```python
from build123d import *

# Parameters (mm, degrees)
BOSS_EXTRUDE1_DEPTH = 2.5
SKETCH2_R           = 2.5
SKETCH2_R_2         = 7.5
CUT_EXTRUDE1_DEPTH  = 63.69968102
SKETCH4_W           = 10
SKETCH4_H           = 10
CUT_EXTRUDE3_DEPTH  = 10


with BuildPart() as part:
    # Sketch1 → Boss-Extrude1 (new, symmetric)
    with BuildSketch(Plane.XY):
        with BuildLine():
            Line((-40, -37.5), (40, -37.5))
            ThreePointArc((40, -37.5), (47.071067812, -34.571067812), (50, -27.5))
            Line((50, -27.5), (50, 27.5))
            ThreePointArc((50, 27.5), (47.071067812, 34.571067812), (40, 37.5))
            Line((40, 37.5), (-40, 37.5))
            ThreePointArc((-40, 37.5), (-47.071067812, 34.571067812), (-50, 27.5))
            Line((-50, 27.5), (-50, -27.5))
            ThreePointArc((-50, -27.5), (-47.071067812, -34.571067812), (-40, -37.5))
        make_face()
    extrude(amount=BOSS_EXTRUDE1_DEPTH, both=True)

    # Sketch2 → Cut-Extrude1 (cut, through all)
    with BuildSketch(Plane.XY.offset(2.5)):
        with Locations((40, 25)):
            Circle(SKETCH2_R)
        with Locations((-40, 25)):
            Circle(SKETCH2_R)
        with Locations((-40, -25)):
            Circle(SKETCH2_R)
        with Locations((40, -25)):
            Circle(SKETCH2_R)
        Circle(SKETCH2_R_2)
    extrude(amount=-CUT_EXTRUDE1_DEPTH, mode=Mode.SUBTRACT)

    # Sketch4 → Cut-Extrude3 (cut)
    with BuildSketch(Plane(origin=(0, 0, -2.5), x_dir=(-1, 0, 0), z_dir=(0, 0, -1))):
        with Locations((45, 0)):
            Rectangle(SKETCH4_W, SKETCH4_H)
        with Locations((-45, 0)):
            Rectangle(SKETCH4_W, SKETCH4_H)
    extrude(amount=-CUT_EXTRUDE3_DEPTH, mode=Mode.SUBTRACT)


solid = part.part
```
Model file for the job. Use its own axes, mm. A direction names the side the tool comes from. Give positions to 0.01 mm unless a question says otherwise; leave off trailing zeros. Write each loop counter-clockwise with the first axis right and the second up, starting at its lowest first coordinate (ties: lowest second). Pieces come first, ordered by that corner, then holes. Notation, with made-up numbers: (57, 86.5) -> (70, 86.5) arc R12 ccw to (70, 101.5) -> close; hole circle Ø3 at (-29.5, 46.5). An arc over 180 degrees is marked (long way). Use CSV: the item, a comma, the result in double quotes. Start each with the question number.
1) Cut at D-D on y = 0. List the corners of the cut face in (x, z), plus the area to 3 significant figures.
2) Cut at B-B on z = 0.5. List the corners of the cut face in (x, y).
3) Drill centre lines: L1, parallel to Y at x = 0, z = 1.4; L2, parallel to X at y = -23.5, z = 1.6; L3, parallel to X at y = 23, z = -1.9. Where is each one in solid material? Low to high.
4) Cut at A-A on x = 6. List the corners of the cut face in (y, z), plus the area to 3 significant figures.
5) Tool access for faces 5 (the flat face through (-45, 5, 0)), 6 (the flat face through (45, 5, 0)), 7 (the flat face through (-50, 16, 0)): list every direction of +Z, -Z, +X, -X, +Y, -Y with a clear straight run to the whole face (end or side of a thin tool).
6) Cut at C-C on y = -25. List the corners of the cut face in (x, z).
7) Pin check, flat tips, straight feed: P1, Ø12, axis at x = 0, y = 0, coming from the +Z side; P2, Ø2.5, axis at y = 0, z = 0.5, coming from the +X side; P3, Ø1.5, axis at y = 2.5, z = -1, coming from the -X side. Stop position of each tip, or through.
8) Two-plate mould, pull along Y, no slides. Class faces 1 (the cylindrical face through (-46.99, 34.65, 0.04)), 2 (the cylindrical face through (46.99, -34.65, 0.04)), 3 (the cylindrical face through (-38.66, -22.89, 0.04)), 4 (the flat face through (-1, 9, 2.5)): released by +Y, released by -Y, zero draft, split by the parting line, or undercut.
Final values:
1,outline,"(-40, -2.5) -> (-7.5, -2.5) -> (-7.5, 2.5) -> (-40, 2.5) -> close; (7.5, -2.5) -> (40, -2.5) -> (40, 2.5) -> (7.5, 2.5) -> close"
1,area,"325 mm2"
2,outline,"(-50, -27.5) arc R10 ccw to (-40, -37.5) -> (40, -37.5) arc R10 ccw to (50, -27.5) -> (50, -5) -> (40, -5) -> (40, 5) -> (50, 5) -> (50, 27.5) arc R10 ccw to (40, 37.5) -> (-40, 37.5) arc R10 ccw to (-50, 27.5) -> (-50, 5) -> (-40, 5) -> (-40, -5) -> (-50, -5) -> close; hole circle Ø5 at (-40, -25); hole circle Ø5 at (-40, 25); hole circle Ø15 at (0, 0); hole circle Ø5 at (40, -25); hole circle Ø5 at (40, 25)"
3,L1,"y = -37.5 to -7.5, 7.5 to 37.5"
3,L2,"x = -50 to -42, -38 to 38, 42 to 50"
3,L3,"x = -50 to -41.5, -38.5 to 38.5, 41.5 to 50"
4,outline,"(-37.5, -2.5) -> (-4.5, -2.5) -> (-4.5, 2.5) -> (-37.5, 2.5) -> close; (4.5, -2.5) -> (37.5, -2.5) -> (37.5, 2.5) -> (4.5, 2.5) -> close"
4,area,"330 mm2"
5,face 5,"+Z, -Z, -X"
5,face 6,"+Z, -Z, +X"
5,face 7,"+Z, -Z, -X, +Y, -Y"
6,outline,"(-50, -2.5) -> (-42.5, -2.5) -> (-42.5, 2.5) -> (-50, 2.5) -> close; (-37.5, -2.5) -> (37.5, -2.5) -> (37.5, 2.5) -> (-37.5, 2.5) -> close; (42.5, -2.5) -> (50, -2.5) -> (50, 2.5) -> (42.5, 2.5) -> close"
7,P1,"passes through"
7,P2,"stops at x = 40"
7,P3,"stops at x = -40"
8,face 1,"released by +Y"
8,face 2,"released by -Y"
8,face 3,"undercut"
8,face 4,"zero draft"
